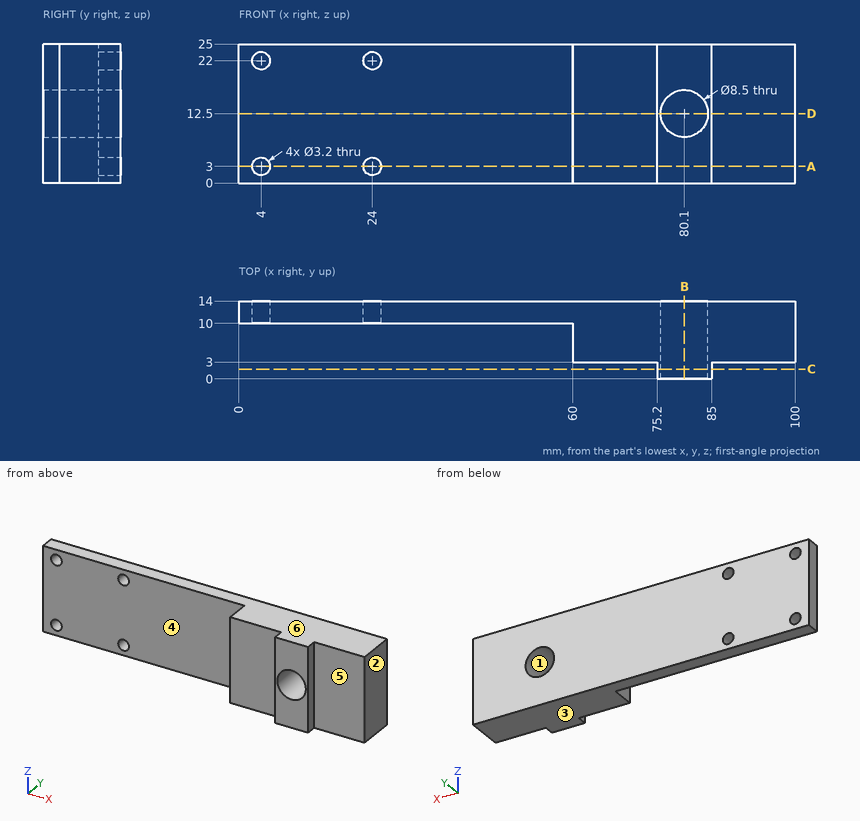
Answer from the drawing. Dimensions are ordinates in mm from the lowest x, y and z of the part. A direction names the side the tool comes from. Give positions to 0.01 mm unless a question says otherwise; leave off trailing zeros. Order: outer loops, then holes, each group sorted by start corner. A loop starts at its lowest first (then second) coordinate and runs counter-clockwise, first axis right, second up. Notation, with made-up numbers: (-24, 64.5) - (23, 64.5) arc R20 ccw to (23, 86.5) - close; hole circle Ø2 at (9.5, 34.25). An arc over 180 degrees is marked (long way). One line per item, written item: value. Start each with the question number.
1) A cutting plane is placed at C-C on y = 1.75. Give the vertices of the cut face in (x, z), then the cut area to 3 significant figures.
2) Find the intervals of material crossed by L1, parallel to Z at x = 4, y = 12.95; L2, parallel to Z at x = 80.1, y = 4.5; L3, parallel to X at y = 9.5, z = 12.25, in increasing order.
3) Given pin 1 Ø5.5 at (y, z) = (7, 17) entering from -X; pin 2 Ø7.5 at (x, z) = (92, 12) entering from -Y; pin 3 Ø1.5 at (y, z) = (2, 10.5) entering from -X, each flat-ended and moving along its own axis, determine where each tip first touches the part or whether it passes through.
4) A cutting plane is placed at A-A on z = 3. Give the vertices of the cut face in (x, y).
5) A cutting plane is placed at D-D on z = 12.5. Give the vertices of the cut face in (x, y).
6) A cutting plane is placed at B-B on x = 80.1. Give the vertices of the cut face in (y, z), then the cut area to 3 significant figures.
7) The mould has two halves that part along X. Classify the marked faces 1, 2 and 3: released by +X, released by -X, zero draft, split by the parting line, or undercut.
8) A tool of negligible diameter and unlimited length cuts with its end or side. For the marked faces 4, 5 and 6, from which of +Z, -Z, +X, -X, +Y, -Y can it reach the whole face along a straight path? Write none if from no direction.
Answer sheet:
1. outline: (75.2, 0) - (85, 0) - (85, 25) - (75.2, 25) - close; hole circle Ø8.5 at (80.1, 12.5)
1. area: 188 mm2
2. L1: z = 0 to 1.4, 4.6 to 20.4, 23.6 to 25
2. L2: z = 0 to 8.25, 16.75 to 25
2. L3: x = 60 to 75.86, 84.34 to 100
3. pin 1: stops at x = 60
3. pin 2: stops at y = 3
3. pin 3: stops at x = 75.2
4. outline: (0, 10) - (2.4, 10) - (2.4, 14) - (0, 14) - close; (5.6, 10) - (22.4, 10) - (22.4, 14) - (5.6, 14) - close; (25.6, 10) - (60, 10) - (60, 3) - (75.2, 3) - (75.2, 0) - (85, 0) - (85, 3) - (100, 3) - (100, 14) - (25.6, 14) - close
5. outline: (0, 10) - (60, 10) - (60, 3) - (75.2, 3) - (75.2, 0) - (75.85, 0) - (75.85, 14) - (0, 14) - close; (84.35, 0) - (85, 0) - (85, 3) - (100, 3) - (100, 14) - (84.35, 14) - close
6. outline: (0, 0) - (14, 0) - (14, 8.25) - (0, 8.25) - close; (0, 16.75) - (14, 16.75) - (14, 25) - (0, 25) - close
6. area: 231 mm2
7. face 1: undercut
7. face 2: released by +X
7. face 3: zero draft
8. face 4: +Z, -Z, -X, -Y
8. face 5: +Z, -Z, +X, -Y
8. face 6: +Z, +X, -X, +Y, -Y
